```python
from build123d import *

# Parameters (mm, degrees)
PAD_DEPTH           = 10
SKETCH001_R         = 2.75
SKETCH001_R_2       = 1.8
SKETCH001_R_3       = 0.875
POCKET_DEPTH        = 15.001
POCKET001_DEPTH     = 3
SKETCH003_R         = 5.1
POCKET002_DEPTH     = 2
SKETCH004_R         = 1.9
PAD001_DEPTH        = 0.2
SKETCH005_R         = 2.95
PAD002_DEPTH        = 0.2
PAD003_DEPTH        = 0.2
LINEARPATTERN_COUNT = 6
LINEARPATTERN_PITCH = 3.96
POCKET003_DEPTH     = 2
CHAMFER_SIZE        = 5
CHAMFER001_SIZE     = 0.8


with BuildPart() as part:
    # Sketch → Pad (new body, symmetric)
    with BuildSketch(Plane.XZ):
        with BuildLine():
            ThreePointArc((3.976179, 8.9), (-4.068927, 7.396182), (4.1, 7.9))
            Line((4.1, 7.9), (8.5, 7.9))
            Line((8.5, 7.9), (10, 6.4))
            Line((10, 6.4), (10, 5))
            Line((10, 5), (42, 5))
            Line((42, 5), (42, 0))
            Line((-20, 0), (42, 0))
            Line((-20, 0), (-20, 5))
            Line((-20, 5), (-8, 5))
            Line((-8, 5), (-8, 10))
            ThreePointArc((-3, 15), (-6.535534, 13.535534), (-8, 10))
            Line((-3, 15), (10, 15))
            Line((10, 15), (10, 10.4))
            Line((8.5, 8.9), (10, 10.4))
            Line((8.5, 8.9), (3.976179, 8.9))
        make_face()
    extrude(amount=PAD_DEPTH, both=True)

    # Sketch001 → Pocket (cut, through all)
    with BuildSketch(Plane(origin=(0, 0, 0), x_dir=(1, 0, 0), z_dir=(0, 0, -1))):
        with Locations((-14, 0)):
            Circle(SKETCH001_R)
        with Locations((36, 0)):
            Circle(SKETCH001_R)
        with Locations((6.5, 0)):
            Circle(SKETCH001_R_2)
        with Locations((15.5, -3.8)):
            Circle(SKETCH001_R_3)
        with Locations((25, -3.8)):
            Circle(SKETCH001_R_3)
    extrude(amount=-POCKET_DEPTH, mode=Mode.SUBTRACT)

    # Sketch002 → Pocket001 (cut)
    with BuildSketch(Plane(origin=(0, 0, 0), x_dir=(1, 0, 0), z_dir=(0, 0, -1))):
        Polygon((6.5, 3.406367), (3.55, 1.703183), (3.55, -1.703183), (6.5, -3.406367), (9.45, -1.703183), (9.45, 1.703183), align=None)
    extrude(amount=-POCKET001_DEPTH, mode=Mode.SUBTRACT)

    # Sketch003 → Pocket002 (cut)
    with BuildSketch(Plane.XY.offset(5)):
        with Locations((36, 0)):
            Circle(SKETCH003_R)
        with Locations((-14, 0)):
            Circle(SKETCH003_R)
    extrude(amount=-POCKET002_DEPTH, mode=Mode.SUBTRACT)

    # Sketch004 → Pad001 (join)
    with BuildSketch(Plane.XY.offset(8.9)):
        with Locations((6.5, 0)):
            Circle(SKETCH004_R)
    extrude(amount=PAD001_DEPTH)

    # Sketch005 → Pad002 (join)
    with BuildSketch(Plane.XY.offset(3)):
        with Locations((6.5, 0)):
            Circle(SKETCH005_R)
    extrude(amount=PAD002_DEPTH)

    # Sketch006 → Pad003 (join)
    with BuildSketch(Plane.XZ.offset(-10)):
        with BuildLine():
            ThreePointArc((4.1, 7.9), (4.068927, 8.403818), (3.976179, 8.9))
            Line((8.5, 8.9), (3.976179, 8.9))
            Line((8.5, 7.9), (8.5, 8.9))
            Line((4.1, 7.9), (8.5, 7.9))
        make_face()
    pad003 = extrude(amount=PAD003_DEPTH)

    # LinearPattern: Pad003 ×6
    with Locations(*[(0, -i * LINEARPATTERN_PITCH, 0) for i in range(1, LINEARPATTERN_COUNT)]):
        add(pad003)

    # Sketch007 → Pocket003 (cut)
    with BuildSketch(Plane.XY.offset(15)):
        with BuildLine():
            ThreePointArc((6.5, 3.65), (2.85, 0), (6.5, -3.65))
            Line((10.5, -3.65), (6.5, -3.65))
            Line((10.5, 3.65), (10.5, -3.65))
            Line((6.5, 3.65), (10.5, 3.65))
        make_face()
    extrude(amount=-POCKET003_DEPTH, mode=Mode.SUBTRACT)

    # Chamfer
    chamfer_edges = [part.edges().sort_by_distance(p)[0] for p in [
        (-20, -10, 2.5),
        (42, -10, 2.5),
        (42, 10, 2.5),
        (-20, 10, 2.5),
    ]]
    chamfer(chamfer_edges, length=CHAMFER_SIZE)

    # Chamfer001
    chamfer001_edges = [part.edges().sort_by_distance(p)[0] for p in [
        (-8, -10, 7.5),
        (-6.535534, -10, 13.535534),
        (3.5, -10, 15),
        (3.5, 10, 15),
        (-6.535534, 10, 13.535534),
        (-8, 10, 7.5),
    ]]
    chamfer(chamfer001_edges, length=CHAMFER001_SIZE)


solid = part.part
```
Geometry check sheet. Reference: the model listing, model coordinates, mm. A direction names the side the tool comes from. Round coordinates to 2 decimals unless told otherwise and drop trailing zeros. Loops run counter-clockwise (first coordinate to the right, second up) from the corner with the lowest first, then second, coordinate; pieces in that order, holes last. Notation, with made-up numbers: (14.5, 85.5) -> (43.5, 85.5) arc R21 cw to (43.5, 101.5) -> close; hole circle Ø11 at (-10, -11.5). An arc over 180 degrees is marked (long way). Use a Markdown table: item, result.
(1) Sectioned sample at B-B (z = 1.5). Enter the section's corners in (x, y) (3 decimals).
Calculated:
| item | result |
|---|---|
| outline | (-20, -5) -> (-15, -10) -> (37, -10) -> (42, -5) -> (42, 5) -> (37, 10) -> (-15, 10) -> (-20, 5) -> close; hole circle Ø5.5 at (-14, 0); hole (3.55, -1.703) -> (6.5, -3.406) -> (9.45, -1.703) -> (9.45, 1.703) -> (6.5, 3.406) -> (3.55, 1.703) -> close; hole circle Ø1.75 at (15.5, 3.8); hole circle Ø1.75 at (25, 3.8); hole circle Ø5.5 at (36, 0) |
(2) Sectioned sample at C-C (x = 36). Enter the section's corners in (y, z).
Calculated:
| item | result |
|---|---|
| outline | (-10, 0) -> (-2.75, 0) -> (-2.75, 3) -> (-5.1, 3) -> (-5.1, 5) -> (-10, 5) -> close; (2.75, 0) -> (10, 0) -> (10, 5) -> (5.1, 5) -> (5.1, 3) -> (2.75, 3) -> close |
(3) Scan lines: probe 1 along X at (y, z) = (0, 1.8); probe 2 along Y at (x, z) = (6.5, 5.4); probe 3 along Y at (x, z) = (36, 0.65). Record each from-to range of solid material in increasing order.
Calculated:
| item | result |
|---|---|
| probe 1 | -20 to -16.75, -11.25 to 3.55, 9.45 to 33.25, 38.75 to 42 |
| probe 2 | -10 to -1.8, 1.8 to 10 |
| probe 3 | -10 to -2.75, 2.75 to 10 |
(4) Mould release check, pull along Y, two halves, no side actions. Record for faces 1 (the flat face through (40, 7, 3)), 2 (the cylindrical face through (14.626, 3.762, 2.465)), 3 (the flat face through (6, 4, 8.9)), 4 (the flat face through (-8, 0, 7)): released by +Y, released by -Y, zero draft, split by the parting line, or undercut.
Calculated:
| item | result |
|---|---|
| face 1 | released by +Y |
| face 2 | undercut |
| face 3 | undercut |
| face 4 | zero draft |
(5) Set-up check for faces 5 (the flat face through (9.2, -0.1, 7.2)), 6 (the flat face through (10, 0, 6)), 7 (the flat face through (5.05, -2.57, 1.48)), 8 (the flat face through (6, -8, 7.9)), 9 (the cylindrical face through (8.217, -0.541, 11.023)): record each of +Z, -Z, +X, -X, +Y, -Y from which the full face is reachable in a straight line by a thin tool's end or side.
Calculated:
| item | result |
|---|---|
| face 5 | +X, +Y, -Y |
| face 6 | +Z, +X, +Y, -Y |
| face 7 | -Z |
| face 8 | +X |
| face 9 | +Z |
(6) Go/stop test with flat-tipped pins: P1, Ø1, axis at x = -12.5, y = 6, coming from the +Z side; P2, Ø1.5, axis at y = -7, z = 6, coming from the -X side; P3, Ø1, axis at y = 1, z = 12, coming from the +X side; P4, Ø12, axis at x = 16.5, y = 6.5, coming from the -Z side. Record where each tip stops, or that it passes through.
Calculated:
| item | result |
|---|---|
| P1 | z = 5 |
| P2 | x = -8 |
| P3 | x = 10 |
| P4 | z = 0 |
(7) Sectioned sample at D-D (y = 0). Give the number of separate pieces and of enclosed holes in the cut face, then the cut area to 3 significant figures.
Calculated:
| item | result |
|---|---|
| separate pieces | 3 |
| enclosed holes | 0 |
| area | 287 mm² |
(8) Sectioned sample at A-A (x = 0). Enter the section's corners in (y, z).
Calculated:
| item | result |
|---|---|
| outline | (-10, 0) -> (10, 0) -> (10, 3.8) -> (-10, 3.8) -> close; (-10, 12) -> (10, 12) -> (10, 14.2) -> (9.2, 15) -> (-9.2, 15) -> (-10, 14.2) -> close |
